Geometry: final body of the model. Coordinates: model frame, mm. Face numbers are marked on the shaded views. A direction names the side the tool comes from. Round coordinates to 2 decimals unless told otherwise and drop trailing zeros. Loops run counter-clockwise (first coordinate to the right, second up) from the corner with the lowest first, then second, coordinate; pieces in that order, holes last. Notation, with made-up numbers: M 37.25,72.25 L 63.25,72.25 A22 cw 63.25,97.25 Z; hole C -12.5,-29 d11. An arc over 180 degrees is marked long. Answer as a JSON object with one key per item and string values.
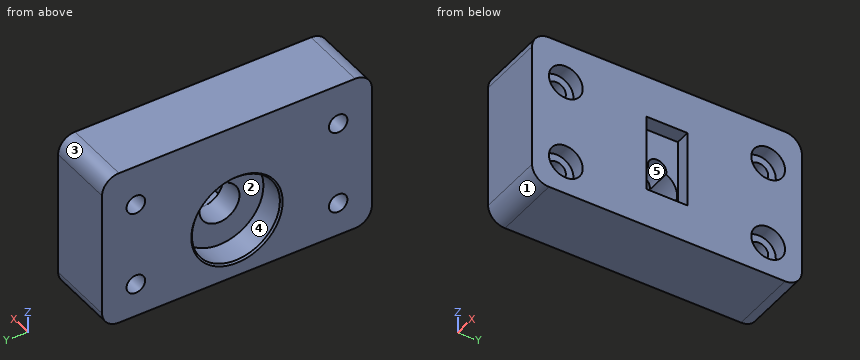
from build123d import *

# Parameters (mm, degrees)
ESQUISSE1_W                                        = 20
ESQUISSE1_H                                        = 80
BOSS_EXTRU_1_DEPTH                                 = 47
ESQUISSE2_R                                        = 13.05
ENL_V_MAT_EXTRU_1_DEPTH                            = 8
ENL_V_MAT_EXTRU_2_REACH                            = 14
CHAMBRAGE_POUR_VIS_T_TE_HEXAGONALE_M52_D           = 5.5
CHAMBRAGE_POUR_VIS_T_TE_HEXAGONALE_M52_CBORE_D     = 10
CHAMBRAGE_POUR_VIS_T_TE_HEXAGONALE_M52_CBORE_DEPTH = 4.2
CONG_1_R                                           = 5
ESQUISSE8_W                                        = 22.8
ESQUISSE8_H                                        = 12.1
ENL_V_MAT_EXTRU_4_DEPTH                            = 4.5
ENL_V_MAT_EXTRU_4_TAPER                            = -1
CHANFREIN1_SIZE                                    = 0.5


with BuildPart() as part:
    # Esquisse1 → Boss.-Extru.1 (new body)
    with BuildSketch(Plane.XY):
        with Locations((10, 40)):
            Rectangle(ESQUISSE1_W, ESQUISSE1_H)
    extrude(amount=BOSS_EXTRU_1_DEPTH)

    # Esquisse2 → Enlèv. mat.-Extru.1 (cut)
    with BuildSketch(Plane.ZY):
        with Locations((17.5, 40)):
            Circle(ESQUISSE2_R)
    extrude(amount=-ENL_V_MAT_EXTRU_1_DEPTH, mode=Mode.SUBTRACT)

    # Esquisse3 → Enlèv. mat.-Extru.2 (cut, up to next)
    with BuildSketch(Plane.ZY.offset(-8), mode=Mode.PRIVATE) as enl_v_mat_extru_2_sk1:
        with BuildLine():
            ThreePointArc((22.825826446, 42.652936611), (11.55, 40), (22.825826446, 37.347063389))
            ThreePointArc((22.825826446, 37.347063389), (26.3, 40), (22.825826446, 42.652936611))
        make_face()
    enl_v_mat_extru_2_tool1 = extrude(enl_v_mat_extru_2_sk1.sketch, amount=-ENL_V_MAT_EXTRU_2_REACH, mode=Mode.PRIVATE) & part.part
    add(enl_v_mat_extru_2_tool1.solids().sort_by_distance((8, 40, 18.266678))[0], mode=Mode.SUBTRACT)

    # Chambrage pour vis à tête hexagonale M52 (through all)
    with Locations(Plane(origin=(20, 0, 0), x_dir=(0, 0, -1), z_dir=(1, 0, 0))):
        with Locations((-10, 70), (-35, 70), (-35, 10), (-10, 10)):
            CounterBoreHole(CHAMBRAGE_POUR_VIS_T_TE_HEXAGONALE_M52_D / 2, CHAMBRAGE_POUR_VIS_T_TE_HEXAGONALE_M52_CBORE_D / 2, CHAMBRAGE_POUR_VIS_T_TE_HEXAGONALE_M52_CBORE_DEPTH)

    # Congé1
    cong_1_edges = [part.edges().sort_by_distance(p)[0] for p in [
        (10, 80, 47),
        (10, 80, 0),
        (10, 0, 0),
        (10, 0, 47),
    ]]
    fillet(cong_1_edges, radius=CONG_1_R)

    # Esquisse8 → Enlèv. mat.-Extru.4 (cut)
    with BuildSketch(Plane(origin=(20, 0, 0), x_dir=(0, 0, -1), z_dir=(1, 0, 0))):
        with Locations((-22.95, 40)):
            Rectangle(ESQUISSE8_W, ESQUISSE8_H)
    extrude(amount=-ENL_V_MAT_EXTRU_4_DEPTH, taper=ENL_V_MAT_EXTRU_4_TAPER, mode=Mode.SUBTRACT)

    # Chanfrein1
    chanfrein1_edges = [part.edges().sort_by_distance(p)[0] for p in [
        (0, 40, 4.45),
    ]]
    chamfer(chanfrein1_edges, length=CHANFREIN1_SIZE)


solid = part.part
1) Section query C-C (y = 6). Return the cut outline in (x, z), and give its area (3 significant figures).
Results:
{"outline": "M 0,0 L 20,0 L 20,7 L 15.8,7 L 15.8,13 L 20,13 L 20,32 L 15.8,32 L 15.8,38 L 20,38 L 20,47 L 0,47 Z", "area": "890 mm2"}
2) Reachability of the marked faces 4 and 5 from +Z, -Z, +X, -X, +Y, -Y: full face, straight path, thin tool, end or side. Return the list, or none.
Results:
{"face 4": "-X", "face 5": "+X, -X"}
3) Section query D-D (z = 10). Count the separate pieces of the cut face and the enclosed holes in it, and give its area (3 significant figures).
Results:
{"separate pieces": "3", "enclosed holes": "0", "area": "1,170 mm2"}
4) Pin query (flat end, axial travel): P1, Ø9, axis at y = 10, z = 35, coming from the +X side; P2, Ø6, axis at y = 39.5, z = 25.5, coming from the +X side; P3, Ø3.5, axis at y = 70, z = 10, coming from the -X side; P4, Ø7, axis at y = 40, z = 23.55, coming from the -X side. Return the tip coordinate at first contact, or that it passes through.
Results:
{"P1": "x = 15.8", "P2": "x = 15.5", "P3": "through", "P4": "x = 8"}
5) Section query B-B (y = 70). Return the cut outline in (x, z), and give its area (3 significant figures).
Results:
{"outline": "M 0,0 L 20,0 L 20,5 L 15.8,5 L 15.8,7.25 L 0,7.25 Z; M 0,12.75 L 15.8,12.75 L 15.8,15 L 20,15 L 20,30 L 15.8,30 L 15.8,32.25 L 0,32.25 Z; M 0,37.75 L 15.8,37.75 L 15.8,40 L 20,40 L 20,47 L 0,47 Z", "area": "682 mm2"}
6) Section query A-A (x = 4). Return the cut outline in (y, z).
Results:
{"outline": "M 0,5 A5 ccw 5,0 L 75,0 A5 ccw 80,5 L 80,42 A5 ccw 75,47 L 5,47 A5 ccw 0,42 Z; hole C 10,10 d5.5; hole C 10,35 d5.5; hole C 40,17.5 d26.1; hole C 70,10 d5.5; hole C 70,35 d5.5"}
7) Pull-direction query (Y, two-part tool) for the marked faces 1, 2 and 3; classes: +Y half, -Y half, draft (parallel to the pull), parting line (faces both ways), or undercut.
Results:
{"face 1": "-Y half", "face 2": "undercut", "face 3": "+Y half"}
8) Ray query, line 1 (Y direction, x = 8, z = 35); line 2 (Y direction, x = 19.1, z = 10); line 3 (Y direction, x = 6.5, z = 17.5). Return the intervals inside material, ascending.
Results:
{"line 1": "0 to 7.25, 12.75 to 67.25, 72.75 to 80", "line 2": "0 to 5, 15 to 65, 75 to 80", "line 3": "0 to 26.95, 53.05 to 80"}
